CAD build for the part. Positions are in the model's coordinates, mm. Give positions to 0.01 mm unless a question says otherwise; leave off trailing zeros. Loops run counter-clockwise (first coordinate to the right, second up) from the corner with the lowest first, then second, coordinate; pieces in that order, holes last. Notation, with made-up numbers: M 19,63 L 27,63 A17 ccw 27,88 Z; hole C 36.5,2 d11. An arc over 180 degrees is marked long. Answer as CSV lines item,"result".
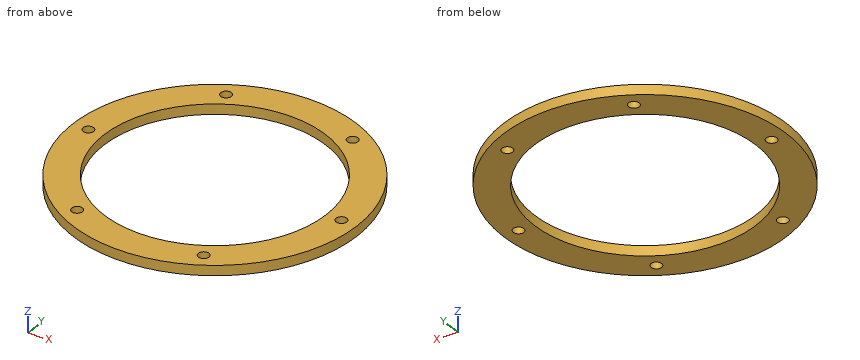
```python
from build123d import *

# Parameters (mm, degrees)
ARO_START         = 69.85
CROQUIS1_R        = 45
CROQUIS1_R_2      = 35.2
ARO_DEPTH         = 3.175
BARRENOS_M3_START = 69.85
CROQUIS2_R        = 1.7
BARRENOS_M3_DEPTH = 3.175


with BuildPart() as part:
    # Croquis1 → Aro (new body)
    with BuildSketch(Plane.XY.offset(ARO_START)):
        Circle(CROQUIS1_R)
        Circle(CROQUIS1_R_2, mode=Mode.SUBTRACT)
    extrude(amount=ARO_DEPTH)

    # Croquis2 → Barrenos_M3 (cut)
    with BuildSketch(Plane.XY.offset(BARRENOS_M3_START)):
        with Locations((40, 0)):
            Circle(CROQUIS2_R)
        with Locations((20, 34.641016151)):
            Circle(CROQUIS2_R)
        with Locations((-20, 34.641016151)):
            Circle(CROQUIS2_R)
        with Locations((-40, 0)):
            Circle(CROQUIS2_R)
        with Locations((-20, -34.641016151)):
            Circle(CROQUIS2_R)
        with Locations((20, -34.641016151)):
            Circle(CROQUIS2_R)
    extrude(amount=BARRENOS_M3_DEPTH, mode=Mode.SUBTRACT)


solid = part.part
```
Q1. Pin check, flat tips, straight feed: P1, Ø1, axis at x = -8, z = 71, coming from the -Y side; P2, Ø4.5, axis at x = 40, y = 0, coming from the +Z side (3 decimals). Stop position of each tip, or through.
Solution:
P1,"stops at y = -44.37"
P2,"stops at z = 73.025"
Q2. Cut at D-D (x = -20). Write the cut outline in (y, z) (3 decimals).
Solution:
outline,"M -40.311,69.85 L -36.341,69.85 L -36.341,73.025 L -40.311,73.025 Z; M -32.941,69.85 L -28.966,69.85 L -28.966,73.025 L -32.941,73.025 Z; M 28.966,69.85 L 32.941,69.85 L 32.941,73.025 L 28.966,73.025 Z; M 36.341,69.85 L 40.311,69.85 L 40.311,73.025 L 36.341,73.025 Z"
Q3. Cut at C-C (z = 70.4). Write the cut outline in (x, y), and give its area (3 significant figures).
Solution:
outline,"C 0,0 d90; hole C -40,0 d3.4; hole C 0,0 d70.4; hole C -20,-34.64 d3.4; hole C -20,34.64 d3.4; hole C 20,-34.64 d3.4; hole C 20,34.64 d3.4; hole C 40,0 d3.4"
area,"2,410 mm²"
Q4. Cut at A-A (x = 0). Write the cut outline in (y, z) (3 decimals).
Solution:
outline,"M -45,69.85 L -35.2,69.85 L -35.2,73.025 L -45,73.025 Z; M 35.2,69.85 L 45,69.85 L 45,73.025 L 35.2,73.025 Z"
Q5. Cut at B-B (y = 0). Write the cut outline in (x, z) (3 decimals).
Solution:
outline,"M -45,69.85 L -41.7,69.85 L -41.7,73.025 L -45,73.025 Z; M -38.3,69.85 L -35.2,69.85 L -35.2,73.025 L -38.3,73.025 Z; M 35.2,69.85 L 38.3,69.85 L 38.3,73.025 L 35.2,73.025 Z; M 41.7,69.85 L 45,69.85 L 45,73.025 L 41.7,73.025 Z"
Q6. Wall check: line 1 (Y direction, x = 0, z = 72.4); line 2 (X direction, y = 36, z = 72.05); line 3 (Y direction, x = 18.5, z = 70.7). Give the ranges that are in metal, low to high. Write a range as [from, to].
Solution:
line 1,"y = [-45, -35.2], [35.2, 45]"
line 2,"x = [-27, -21.02], [-18.98, 18.98], [21.02, 27]"
line 3,"y = [-41.02, -35.44], [-33.84, -29.95], [29.95, 33.84], [35.44, 41.02]"
